Verification items for the finished model (mm, model axes). A direction names the side the tool comes from. Round coordinates to 2 decimals unless told otherwise and drop trailing zeros. Write each loop counter-clockwise with the first axis right and the second up, starting at its lowest first coordinate (ties: lowest second). Pieces come first, ordered by that corner, then holes. Notation, with made-up numbers: (64.5, -37.75) - (91.5, -37.75) arc R18 ccw to (91.5, -16.75) - close; hole circle Ø8 at (1, 70.25). An arc over 180 degrees is marked (long way). Write each question's results on one line, items separated by ' | '.
```python
from build123d import *

# Parameters (mm, degrees)
SKETCH1_R               = 3.4036
BOSS_EXTRUDE1_DEPTH     = 380
SKETCH2_W               = 605.6
SKETCH2_H               = 40
CUT_EXTRUDE1_DEPTH      = 65
CUT_EXTRUDE1_DEPTH_BACK = 71


with BuildPart() as part:
    # Sketch1 → Boss-Extrude1 (new body, symmetric)
    with BuildSketch(Plane.XY):
        with BuildLine():
            Line((-20, 16.952), (-20, 4.7625))
            ThreePointArc((-20, 4.7625), (-19.776815367, 4.223684633), (-19.238, 4.0005))
            Line((-19.238, 4.0005), (-16.2662, 4.0005))
            ThreePointArc((-16.2662, 4.0005), (-15.727384633, 4.223684633), (-15.5042, 4.7625))
            Line((-15.5042, 4.7625), (-15.5042, 10.2235))
            ThreePointArc((-15.5042, 10.2235), (-15.033804775, 10.927496204), (-14.203384633, 10.762315367))
            Line((-14.203384633, 10.762315367), (-8.635059555, 5.19399029))
            ThreePointArc((-8.635059555, 5.19399029), (-7.985348265, 4.221628629), (-7.7572, 3.074649845))
            Line((-7.7572, 3.074649845), (-7.7572, -3.074649845))
            ThreePointArc((-7.7572, -3.074649845), (-7.985348265, -4.221628629), (-8.635059555, -5.19399029))
            Line((-8.635059555, -5.19399029), (-14.203384633, -10.762315367))
            ThreePointArc((-14.203384633, -10.762315367), (-15.033804775, -10.927496204), (-15.5042, -10.2235))
            Line((-15.5042, -10.2235), (-15.5042, -4.7625))
            ThreePointArc((-15.5042, -4.7625), (-15.727384633, -4.223684633), (-16.2662, -4.0005))
            Line((-16.2662, -4.0005), (-19.238, -4.0005))
            ThreePointArc((-19.238, -4.0005), (-19.776815367, -4.223684633), (-20, -4.7625))
            Line((-20, -4.7625), (-20, -16.952))
            ThreePointArc((-20, -16.952), (-19.107261469, -19.107261469), (-16.952, -20))
            Line((-16.952, -20), (-4.7625, -20))
            ThreePointArc((-4.7625, -20), (-4.223684633, -19.776815367), (-4.0005, -19.238))
            Line((-4.0005, -19.238), (-4.0005, -16.2662))
            ThreePointArc((-4.0005, -16.2662), (-4.223684633, -15.727384633), (-4.7625, -15.5042))
            Line((-4.7625, -15.5042), (-10.2235, -15.5042))
            ThreePointArc((-10.2235, -15.5042), (-10.927496204, -15.033804775), (-10.762315367, -14.203384633))
            Line((-10.762315367, -14.203384633), (-5.19399029, -8.635059555))
            ThreePointArc((-5.19399029, -8.635059555), (-4.221628629, -7.985348265), (-3.074649845, -7.7572))
            Line((-3.074649845, -7.7572), (3.074649845, -7.7572))
            ThreePointArc((3.074649845, -7.7572), (4.221628629, -7.985348265), (5.19399029, -8.635059555))
            Line((5.19399029, -8.635059555), (10.762315367, -14.203384633))
            ThreePointArc((10.762315367, -14.203384633), (10.927496204, -15.033804775), (10.2235, -15.5042))
            Line((10.2235, -15.5042), (4.7625, -15.5042))
            ThreePointArc((4.7625, -15.5042), (4.223684633, -15.727384633), (4.0005, -16.2662))
            Line((4.0005, -16.2662), (4.0005, -19.238))
            ThreePointArc((4.0005, -19.238), (4.223684633, -19.776815367), (4.7625, -20))
            Line((4.7625, -20), (16.952, -20))
            ThreePointArc((16.952, -20), (19.107261469, -19.107261469), (20, -16.952))
            Line((20, -16.952), (20, -4.7625))
            ThreePointArc((20, -4.7625), (19.776815367, -4.223684633), (19.238, -4.0005))
            Line((19.238, -4.0005), (16.2662, -4.0005))
            ThreePointArc((16.2662, -4.0005), (15.727384633, -4.223684633), (15.5042, -4.7625))
            Line((15.5042, -4.7625), (15.5042, -10.2235))
            ThreePointArc((15.5042, -10.2235), (15.033804775, -10.927496204), (14.203384633, -10.762315367))
            Line((14.203384633, -10.762315367), (8.635059555, -5.19399029))
            ThreePointArc((8.635059555, -5.19399029), (7.985348265, -4.221628629), (7.7572, -3.074649845))
            Line((7.7572, -3.074649845), (7.7572, 3.074649845))
            ThreePointArc((7.7572, 3.074649845), (7.985348265, 4.221628629), (8.635059555, 5.19399029))
            Line((8.635059555, 5.19399029), (14.203384633, 10.762315367))
            ThreePointArc((14.203384633, 10.762315367), (15.033804775, 10.927496204), (15.5042, 10.2235))
            Line((15.5042, 10.2235), (15.5042, 4.7625))
            ThreePointArc((15.5042, 4.7625), (15.727384633, 4.223684633), (16.2662, 4.0005))
            Line((16.2662, 4.0005), (19.238, 4.0005))
            ThreePointArc((19.238, 4.0005), (19.776815367, 4.223684633), (20, 4.7625))
            Line((20, 4.7625), (20, 16.952))
            ThreePointArc((20, 16.952), (19.107261469, 19.107261469), (16.952, 20))
            Line((16.952, 20), (4.7625, 20))
            ThreePointArc((4.7625, 20), (4.223684633, 19.776815367), (4.0005, 19.238))
            Line((4.0005, 19.238), (4.0005, 16.2662))
            ThreePointArc((4.0005, 16.2662), (4.223684633, 15.727384633), (4.7625, 15.5042))
            Line((4.7625, 15.5042), (10.2235, 15.5042))
            ThreePointArc((10.2235, 15.5042), (10.927496204, 15.033804775), (10.762315367, 14.203384633))
            Line((10.762315367, 14.203384633), (5.19399029, 8.635059555))
            ThreePointArc((5.19399029, 8.635059555), (4.221628629, 7.985348265), (3.074649845, 7.7572))
            Line((3.074649845, 7.7572), (-3.074649845, 7.7572))
            ThreePointArc((-3.074649845, 7.7572), (-4.221628629, 7.985348265), (-5.19399029, 8.635059555))
            Line((-5.19399029, 8.635059555), (-10.762315367, 14.203384633))
            ThreePointArc((-10.762315367, 14.203384633), (-10.927496204, 15.033804775), (-10.2235, 15.5042))
            Line((-10.2235, 15.5042), (-4.7625, 15.5042))
            ThreePointArc((-4.7625, 15.5042), (-4.223684633, 15.727384633), (-4.0005, 16.2662))
            Line((-4.0005, 16.2662), (-4.0005, 19.238))
            ThreePointArc((-4.0005, 19.238), (-4.223684633, 19.776815367), (-4.7625, 20))
            Line((-4.7625, 20), (-16.952, 20))
            ThreePointArc((-16.952, 20), (-19.107261469, 19.107261469), (-20, 16.952))
        make_face()
        Circle(SKETCH1_R, mode=Mode.SUBTRACT)
    extrude(amount=BOSS_EXTRUDE1_DEPTH, both=True)

    # Sketch2 → Cut-Extrude1 (cut, two sides)
    with BuildSketch(Plane(origin=(0, 0, 0), x_dir=(0, 0, -1), z_dir=(1, 0, 0))) as cut_extrude1_sk:
        with Locations((77.2, 0)):
            Rectangle(SKETCH2_W, SKETCH2_H)
    extrude(amount=CUT_EXTRUDE1_DEPTH, mode=Mode.SUBTRACT)
    extrude(cut_extrude1_sk.sketch, amount=-CUT_EXTRUDE1_DEPTH_BACK, mode=Mode.SUBTRACT)


solid = part.part
```
(1) Go/stop test with flat-tipped pins: pin 1 Ø1.5 at (y, z) = (18.5, 302) entering from -X; pin 2 Ø1.8 at (y, z) = (-1, 333.5) entering from -X; pin 3 Ø7 at (x, z) = (1, 281.5) entering from +Y. Record where each tip stops, or that it passes through.
Answer:
pin 1: x = -19.89 | pin 2: x = -7.76 | pin 3: y = 19.95
(2) Section check A-A (y = 0). Record the cut outline in (x, z).
Answer:
outline: (-7.76, 225.6) - (-3.4, 225.6) - (-3.4, 380) - (-7.76, 380) - close; (3.4, 225.6) - (7.76, 225.6) - (7.76, 380) - (3.4, 380) - close
(3) Mould release check, pull along Y, two halves, no side actions. Record for faces 6 (the flat face through (4, -18, 304)), 7 (the cylindrical face through (-19.083, 19.131, 303.881)), 8 (the flat face through (-11.46, 8.02, 303.88)), 9 (the flat face through (-15.504, -8, 304)): released by +Y, released by -Y, zero draft, split by the parting line, or undercut.
Answer:
face 6: zero draft | face 7: released by +Y | face 8: undercut | face 9: undercut
(4) Thickness scan on L1, parallel to Y at x = 0, z = 314.5; L2, parallel to Y at x = -6.5, z = 335.5; L3, parallel to X at y = -5.5, z = 294.5. Record the ranges inside material, lowest first.
Answer:
L1: -7.76 to -3.4, 3.4 to 7.76 | L2: -20 to -15.5, -9.94 to 9.94, 15.5 to 20 | L3: -20 to -15.5, -8.94 to 8.94, 15.5 to 20
(5) Set-up check for faces 1 (the flat face through (18, 4, 304)), 2 (the flat face through (-7.94, 11.38, 303.88)), 3 (the flat face through (-18, -4, 304)), 4 (the flat face through (4, 18, 304)), 5 (the flat face through (11, -20, 304)): record each of +Z, -Z, +X, -X, +Y, -Y from which the full face is reachable in a straight line by a thin tool's end or side.
Answer:
face 1: +Z, -Z, +X | face 2: +Z, -Z | face 3: +Z, -Z, -X | face 4: +Z, -Z, +Y | face 5: +Z, -Z, +X, -X, -Y
